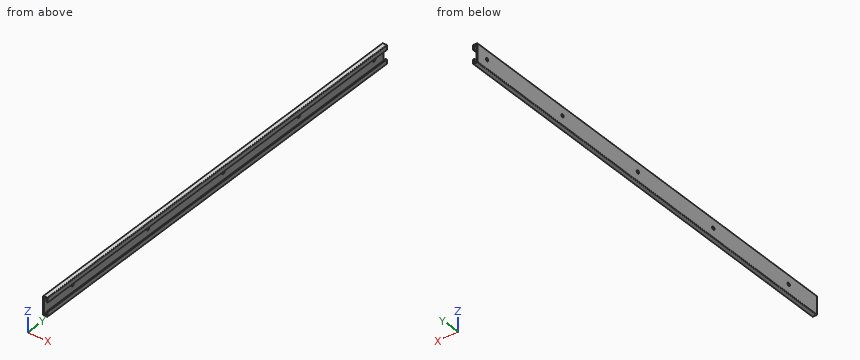
from build123d import *

# Parameters (mm, degrees)
BOSS_EXTRUDE1_DEPTH = 914.4
CUT_EXTRUDE1_REACH  = 4.54
SKETCH2_R           = 3.175


with BuildPart() as part:
    # Sketch1 → Boss-Extrude1 (new body)
    with BuildSketch(Plane(origin=(0, 0, 0), x_dir=(1, 0, 0), z_dir=(0, 1, 0))):
        with BuildLine():
            Line((9.525, 34.29), (9.525, 26.035))
            Line((9.525, 26.035), (6.985, 26.035))
            Line((6.985, 26.035), (6.985, 33.02))
            Line((6.985, 33.02), (2.54, 33.02))
            Line((2.54, 33.02), (2.54, 0))
            Line((2.54, 0), (6.985, 0))
            Line((6.985, 0), (6.985, 6.985))
            Line((6.985, 6.985), (9.525, 6.985))
            Line((9.525, 6.985), (9.525, -1.27))
            ThreePointArc((9.525, -1.27), (9.153025612, -2.168025612), (8.255, -2.54))
            Line((8.255, -2.54), (1.27, -2.54))
            ThreePointArc((1.27, -2.54), (0.371974388, -2.168025612), (0, -1.27))
            Line((0, -1.27), (0, 34.29))
            ThreePointArc((0, 34.29), (0.371974388, 35.188025612), (1.27, 35.56))
            Line((1.27, 35.56), (8.255, 35.56))
            ThreePointArc((8.255, 35.56), (9.153025612, 35.188025612), (9.525, 34.29))
        make_face()
    extrude(amount=BOSS_EXTRUDE1_DEPTH)

    # Sketch2 → Cut-Extrude1 (cut, up to next)
    with BuildSketch(Plane(origin=(2.54, 0, 0), x_dir=(0, 0, -1), z_dir=(1, 0, 0)), mode=Mode.PRIVATE) as cut_extrude1_sk1:
        with Locations((16.51, 76.2)):
            Circle(SKETCH2_R)
    cut_extrude1_tool1 = extrude(cut_extrude1_sk1.sketch, amount=-CUT_EXTRUDE1_REACH, mode=Mode.PRIVATE) & part.part
    add(cut_extrude1_tool1.solids().sort_by_distance((2.54, 76.2, -16.51))[0], mode=Mode.SUBTRACT)
    # Sketch2 → Cut-Extrude1 (cut, up to next)
    with BuildSketch(Plane(origin=(2.54, 0, 0), x_dir=(0, 0, -1), z_dir=(1, 0, 0)), mode=Mode.PRIVATE) as cut_extrude1_sk2:
        with Locations((16.51, 279.4)):
            Circle(SKETCH2_R)
    cut_extrude1_tool2 = extrude(cut_extrude1_sk2.sketch, amount=-CUT_EXTRUDE1_REACH, mode=Mode.PRIVATE) & part.part
    add(cut_extrude1_tool2.solids().sort_by_distance((2.54, 279.4, -16.51))[0], mode=Mode.SUBTRACT)
    # Sketch2 → Cut-Extrude1 (cut, up to next)
    with BuildSketch(Plane(origin=(2.54, 0, 0), x_dir=(0, 0, -1), z_dir=(1, 0, 0)), mode=Mode.PRIVATE) as cut_extrude1_sk3:
        with Locations((16.51, 482.6)):
            Circle(SKETCH2_R)
    cut_extrude1_tool3 = extrude(cut_extrude1_sk3.sketch, amount=-CUT_EXTRUDE1_REACH, mode=Mode.PRIVATE) & part.part
    add(cut_extrude1_tool3.solids().sort_by_distance((2.54, 482.6, -16.51))[0], mode=Mode.SUBTRACT)
    # Sketch2 → Cut-Extrude1 (cut, up to next)
    with BuildSketch(Plane(origin=(2.54, 0, 0), x_dir=(0, 0, -1), z_dir=(1, 0, 0)), mode=Mode.PRIVATE) as cut_extrude1_sk4:
        with Locations((16.51, 685.8)):
            Circle(SKETCH2_R)
    cut_extrude1_tool4 = extrude(cut_extrude1_sk4.sketch, amount=-CUT_EXTRUDE1_REACH, mode=Mode.PRIVATE) & part.part
    add(cut_extrude1_tool4.solids().sort_by_distance((2.54, 685.8, -16.51))[0], mode=Mode.SUBTRACT)
    # Sketch2 → Cut-Extrude1 (cut, up to next)
    with BuildSketch(Plane(origin=(2.54, 0, 0), x_dir=(0, 0, -1), z_dir=(1, 0, 0)), mode=Mode.PRIVATE) as cut_extrude1_sk5:
        with Locations((16.51, 889)):
            Circle(SKETCH2_R)
    cut_extrude1_tool5 = extrude(cut_extrude1_sk5.sketch, amount=-CUT_EXTRUDE1_REACH, mode=Mode.PRIVATE) & part.part
    add(cut_extrude1_tool5.solids().sort_by_distance((2.54, 889, -16.51))[0], mode=Mode.SUBTRACT)


solid = part.part
Model file for the job. Use its own axes, mm. Coordinates: 2 decimals unless noted, no trailing zeros. Write each loop counter-clockwise with the first axis right and the second up, starting at its lowest first coordinate (ties: lowest second). Pieces come first, ordered by that corner, then holes. Notation, with made-up numbers: (36.25, 85) -> (83.25, 85) arc R22 ccw to (83.25, 117) -> close; hole circle Ø1 at (50.25, 34.25). An arc over 180 degrees is marked (long way). One line per item, written item: value. Start each with the question number.
1) Probe probe 1 along Y at (x, z) = (1.35, -16.51) (3 decimals); probe 2 along X at (y, z) = (161, -2.5) (3 decimals); probe 3 along Z at (x, y) = (1.55, 482.6) (3 decimals). List the from-to ranges inside material, lowest first.
2) Flat gauge pins, fed straight in: pin 1 Ø5 at (y, z) = (685.8, -16.51) entering from +X; pin 2 Ø8.5 at (y, z) = (279.4, -16.51) entering from +X. Where does each tip first touch, or does it go through?
3) Slice it at A-A on y = 350. Write the cut outline in (x, z) (3 decimals), then the cut area to 3 significant figures.
Answers follow:
1. probe 1: 0 to 73.025, 79.375 to 276.225, 282.575 to 479.425, 485.775 to 682.625, 688.975 to 885.825, 892.175 to 914.4
1. probe 2: 0 to 2.54, 6.985 to 9.525
1. probe 3: -35.56 to -19.685, -13.335 to 2.54
2. pin 1: through
2. pin 2: x = 2.54
3. outline: (0, -34.29) arc R1.27 ccw to (1.27, -35.56) -> (8.255, -35.56) arc R1.27 ccw to (9.525, -34.29) -> (9.525, -26.035) -> (6.985, -26.035) -> (6.985, -33.02) -> (2.54, -33.02) -> (2.54, 0) -> (6.985, 0) -> (6.985, -6.985) -> (9.525, -6.985) -> (9.525, 1.27) arc R1.27 ccw to (8.255, 2.54) -> (1.27, 2.54) arc R1.27 ccw to (0, 1.27) -> close
3. area: 166 mm2
